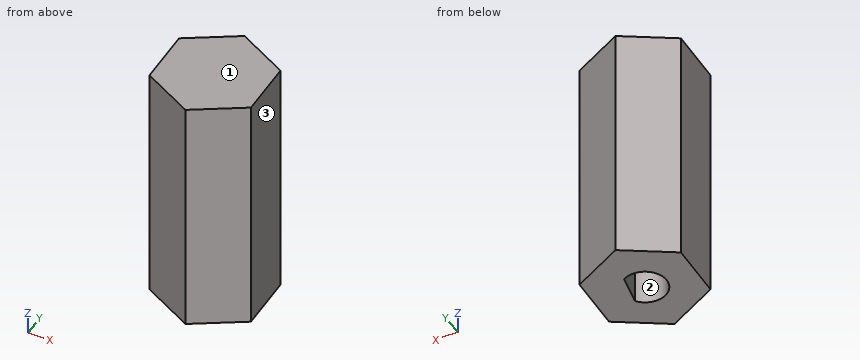
```python
from build123d import *

# Parameters (mm, degrees)
BOSS_EXTRUDE1_DEPTH = 17
CUT_EXTRUDE7_DEPTH  = 8


with BuildPart() as part:
    # Sketch1 → Boss-Extrude1 (new body)
    with BuildSketch(Plane.XY):
        Polygon((3.574198426, -1.886382503), (3.420754381, 2.152155384), (-0.153444044, 4.038537886), (-3.574198426, 1.886382503), (-3.420754381, -2.152155384), (0.153444044, -4.038537886), align=None)
    extrude(amount=BOSS_EXTRUDE1_DEPTH)

    # Sketch2 → Cut-Extrude7 (cut)
    with BuildSketch(Plane.XY):
        with BuildLine():
            Line((0.76003439, 1.293192842), (1.195356952, -0.906157689))
            ThreePointArc((1.195356952, -0.906157689), (-1.471453198, -0.291248151), (0.76003439, 1.293192842))
        make_face()
    extrude(amount=CUT_EXTRUDE7_DEPTH, mode=Mode.SUBTRACT)


solid = part.part
```
Verification items for the finished model (mm, model axes). Face numbers are marked on the shaded views. Round coordinates to 2 decimals unless told otherwise and drop trailing zeros. Loops run counter-clockwise (first coordinate to the right, second up) from the corner with the lowest first, then second, coordinate; pieces in that order, holes last. Notation, with made-up numbers: (84.25, 27) -> (109.25, 27) arc R18 ccw to (109.25, 43) -> close; hole circle Ø7 at (-5, 28.25). An arc over 180 degrees is marked (long way). Answer as a JSON object with one key per item and string values.
Q1. Section check D-D (x = 1). Record the boundary of the cut face in (y, z).
Data:
{"outline": "(-3.51, 0) -> (-1.12, 0) -> (-1.12, 8) -> (0.08, 8) -> (0.08, 0) -> (3.43, 0) -> (3.43, 17) -> (-3.51, 17) -> close"}
Q2. Go/stop test with a flat-tipped pin: P1, Ø1.5, axis at x = 2, z = 5.5, coming from the -Y side. Record where the tip stops, or that it passes through.
Data:
{"P1": "stops at y = -3.35"}
Q3. Draft check along Y on the marked faces 1, 2 and 3. Enter one of: pulls with the +Y half, pulls with the -Y half, needs draft (parallel to the pull), parting line crosses it, or undercut.
Data:
{"face 1": "needs draft", "face 2": "undercut", "face 3": "pulls with the +Y half"}
Q4. Section check A-A (z = 2.5). Record the boundary of the cut face in (x, y).
Data:
{"outline": "(-3.57, 1.89) -> (-3.42, -2.15) -> (0.15, -4.04) -> (3.57, -1.89) -> (3.42, 2.15) -> (-0.15, 4.04) -> close; hole (0.76, 1.29) arc R1.5 ccw (long way) to (1.2, -0.91) -> close"}
Q5. Section check B-B (z = 14.5). Record the boundary of the cut face in (x, y), then the cut area to 3 significant figures.
Data:
{"outline": "(-3.57, 1.89) -> (-3.42, -2.15) -> (0.15, -4.04) -> (3.57, -1.89) -> (3.42, 2.15) -> (-0.15, 4.04) -> close", "area": "42.4 mm2"}
Q6. Section check C-C (y = 0.75). Record the boundary of the cut face in (x, z), then the cut area to 3 significant figures.
Data:
{"outline": "(-3.53, 0) -> (-1.3, 0) -> (-1.3, 8) -> (0.87, 8) -> (0.87, 0) -> (3.47, 0) -> (3.47, 17) -> (-3.53, 17) -> close", "area": "102 mm2"}
Q7. Scan lines: line 1 (Z direction, x = -1, y = -0.75); line 2 (X direction, y = 0, z = 5.75); line 3 (Y direction, x = 0, z = 1.5). Record each from-to range of solid material in increasing order. Write a range as from..to.
Data:
{"line 1": "z = 8..17", "line 2": "x = -3.5..-1.5, 1.02..3.5", "line 3": "y = -3.96..-1.5, 1.5..3.96"}
